from build123d import *

# Parameters (mm, degrees)
F0_R     = 38.288437
F0_R_2   = 4.4069
F1_DEPTH = 6.35


with BuildPart() as f1:
    # F0 (on Top) → F1 (new body)
    with BuildSketch(Plane.XY):
        with BuildLine():
            ThreePointArc((12.395513, 51.224059), (0.470607, 56.227106), (-11.454299, 51.224059))
            Line((-11.454299, 51.224059), (-32.375696, 29.918984))
            ThreePointArc((-32.375696, 29.918984), (-46.92978, -5.660917), (-32.394285, -41.248415))
            Line((-32.394285, -41.248415), (-11.460414, -62.588481))
            ThreePointArc((-11.460414, -62.588481), (0.470607, -67.597759), (12.401629, -62.588481))
            Line((12.401629, -62.588481), (33.335499, -41.248415))
            ThreePointArc((33.335499, -41.248415), (47.870994, -5.660917), (33.31691, 29.918984))
            Line((33.31691, 29.918984), (12.395513, 51.224059))
        make_face()
        with BuildLine():
            ThreePointArc((0.470607, -52.150294), (3.62792, -53.458096), (4.935722, -56.615409))
            ThreePointArc((4.935722, -56.615409), (-2.686706, -59.772722), (0.470607, -52.150294))
        make_face(mode=Mode.SUBTRACT)
        with Locations((0.470607, -5.686851)):
            Circle(F0_R, mode=Mode.SUBTRACT)
        with Locations((0.470607, 45.241707)):
            Circle(F0_R_2, mode=Mode.SUBTRACT)
    extrude(amount=F1_DEPTH)


solid = f1.part
Build history of the part. All positions in model axes, mm. Round coordinates to 2 decimals unless told otherwise and drop trailing zeros. Loops run counter-clockwise (first coordinate to the right, second up) from the corner with the lowest first, then second, coordinate; pieces in that order, holes last. Notation, with made-up numbers: (5, -8.5) -> (31, -8.5) arc R11 cw to (31, 5.5) -> close; hole circle Ø5 at (-1.5, 82.25). An arc over 180 degrees is marked (long way). Use CSV: the item, a comma, the result in double quotes. Start each with the question number.
Q1. Flat gauge pins, fed straight in: pin 1 Ø3 at (x, z) = (-8, 4) entering from +Y; pin 2 Ø5.5 at (x, y) = (0.47, -56.62) entering from -Z; pin 3 Ø1 at (y, z) = (-30, 2) entering from +X. Where does each tip first touch, or does it go through?
Q2. Saw through at C-C on x = 2. Give the cut face in (y, z), and give its area (3 significant figures).
Q3. Drill centre lines: L1, parallel to Y at x = -2, z = 2.25; L2, parallel to Y at x = 1, z = 2.5; L3, parallel to Y at x = -23.5, z = 1.25. Where is each one in solid material? Low to high.
Q4. Saw through at A-A on x = -15. Give the cut face in (y, z), and give its area (3 significant figures).
Q5. Saw through at D-D on z = 4.75. Give the cut face in (x, y).
Q6. Saw through at B-B on y = -11. Give the cut face in (x, z).
Q7. Mould opens along X. For faces 1 (the face through (23.003, 40.422, 3.131)), 2 (the face through (0.285, -67.597, 3.131)), 3 (the face through (-0.48, 40.94, 3.13)) say: +X half, -X half, draft (parallel to the pull), parting line (faces both ways), or undercut.
Solutions:
1,pin 1,"stops at y = 54.7"
1,pin 2,"passes through"
1,pin 3,"stops at x = 41.94"
2,outline,"(-67.53, 0) -> (-60.81, 0) -> (-60.81, 6.35) -> (-67.53, 6.35) -> close; (-52.42, 0) -> (-43.94, 0) -> (-43.94, 6.35) -> (-52.42, 6.35) -> close; (32.57, 0) -> (41.11, 0) -> (41.11, 6.35) -> (32.57, 6.35) -> close; (49.37, 0) -> (56.16, 0) -> (56.16, 6.35) -> (49.37, 6.35) -> close"
2,area,"194 mm^2"
3,L1,"y = -67.41 to -60.33, -52.9 to -43.9, 32.52 to 41.59, 48.89 to 56.04"
3,L2,"y = -67.59 to -61.05, -52.18 to -43.97, 32.6 to 40.87, 49.62 to 56.22"
3,L3,"y = -50.32 to -35.54, 24.17 to 38.96"
4,outline,"(-58.98, 0) -> (-40.71, 0) -> (-40.71, 6.35) -> (-58.98, 6.35) -> close; (29.34, 0) -> (47.61, 0) -> (47.61, 6.35) -> (29.34, 6.35) -> close"
4,area,"232 mm^2"
5,outline,"(-32.39, -41.25) -> (-11.46, -62.59) arc R16.71 ccw to (12.4, -62.59) -> (33.34, -41.25) arc R50.8 ccw to (33.32, 29.92) -> (12.4, 51.22) arc R16.71 ccw to (-11.45, 51.22) -> (-32.38, 29.92) arc R50.8 ccw to start; hole circle Ø76.58 at (0.47, -5.69); hole circle Ø8.93 at (0.47, -56.62); hole circle Ø8.81 at (0.47, 45.24)"
6,outline,"(-46.65, 0) -> (-37.45, 0) -> (-37.45, 6.35) -> (-46.65, 6.35) -> close; (38.39, 0) -> (47.59, 0) -> (47.59, 6.35) -> (38.39, 6.35) -> close"
7,face 1,"+X half"
7,face 2,"parting line"
7,face 3,"undercut"
